```python
from build123d import *

# Parameters (mm, degrees)
F0_W     = 138.9888
F0_H     = 419.989
F1_DEPTH = 6.35
F3_D     = 7.874


with BuildPart() as f1:
    # F0 (on Top) → F1 (new body)
    with BuildSketch(Plane.XY):
        with Locations((69.4944, 309.9943)):
            Rectangle(F0_W, F0_H)
        Polygon((0, 619.9886), (0, 519.9888), (138.9888, 519.9888), (759.0028, 519.9888), (897.9916, 519.9888), (897.9916, 619.9886), align=None)
        with Locations((828.4972, 309.9943)):
            Rectangle(F0_W, F0_H)
        Polygon((0, 99.9998), (0, 0), (897.9916, 0), (897.9916, 99.9998), (759.0028, 99.9998), (138.9888, 99.9998), align=None)
    extrude(amount=F1_DEPTH)

    # F3 (through all)
    with Locations(Plane.XY.offset(6.35)):
        with Locations((108.9914, 539.9786), (124.0028, 554.99), (174.0154, 554.99), (124.0028, 579.9836), (224.028, 579.9836), (224.028, 554.99), (274.0406, 554.99), (324.0532, 579.9836), (324.0532, 554.99), (374.0658, 554.99), (424.0784, 579.9836), (424.0784, 554.99), (474.091, 579.9836), (474.091, 554.99), (524.1036, 554.99), (574.1162, 579.9836), (574.1162, 554.99), (624.1288, 554.99), (674.1414, 579.9836), (674.1414, 554.99), (789.0002, 539.9786), (774.1666, 579.9836), (774.1666, 554.99), (724.154, 554.99), (789.0002, 480.1108), (813.9938, 465.074), (789.0002, 130.0226), (813.9938, 145.034), (789.0002, 180.0352), (789.0002, 230.0478), (813.9938, 225.044), (789.0002, 280.0604), (813.9938, 305.054), (789.0002, 330.073), (789.0002, 380.0856), (813.9938, 385.064), (789.0002, 430.0982), (789.0002, 80.01), (774.1666, 64.9986), (774.1666, 40.005), (724.154, 64.9986), (674.1414, 64.9986), (674.1414, 40.005), (83.9978, 465.074), (108.9914, 480.1108), (108.9914, 430.0982), (83.9978, 385.064), (108.9914, 380.0856), (108.9914, 330.073), (83.9978, 305.054), (108.9914, 280.0604), (83.9978, 225.044), (108.9914, 230.0478), (108.9914, 180.0352), (83.9978, 145.034), (108.9914, 130.0226), (108.9914, 80.01), (124.0028, 64.9986), (124.0028, 40.005), (174.0154, 64.9986), (224.028, 40.005), (224.028, 64.9986), (274.0406, 64.9986), (324.0532, 40.005), (324.0532, 64.9986), (374.0658, 64.9986), (424.0784, 64.9986), (424.0784, 40.005), (474.091, 64.9986), (474.091, 40.005), (524.1036, 64.9986), (574.1162, 64.9986), (624.1288, 64.9986), (574.1162, 40.005)):
            Hole(F3_D / 2)


solid = f1.part
```
For this review, take the finished solid that the model builds, in its own axes (mm). Give positions to 0.01 mm unless a question says otherwise; leave off trailing zeros. Write each loop counter-clockwise with the first axis right and the second up, starting at its lowest first coordinate (ties: lowest second). Pieces come first, ordered by that corner, then holes.
Item 1: Insertion check: P1, Ø7, axis at x = 724.15, y = 65, coming from the -Z side. The pin has a flat end and moves straight along its axis. Give the tip position at first contact, or say it passes through.
Item 2: Wall thickness on probe 1 along X at (y, z) = (472.5, 3.5); probe 2 along Y at (x, z) = (201.5, 3); probe 3 along X at (y, z) = (542.5, 5.5): over which ranges is each line inside the solid? List them lowest first.
Item 3: Take a section at B-B (y = 110). Give the boundary of the cut face in (x, z).
Item 4: Take a section at C-C (z = 3). Give the number of separate pieces and of enclosed holes in the cut face, and give its area (3 significant figures).
Item 5: Take a section at A-A (x = 205). Give the boundary of the cut face in (y, z).
Established:
1. P1: passes through
2. probe 1: x = 0 to 138.99, 759 to 897.99
2. probe 2: y = 0 to 100, 519.99 to 619.99
2. probe 3: x = 0 to 105.97, 112.02 to 785.98, 792.02 to 897.99
3. outline: (0, 0) - (138.99, 0) - (138.99, 6.35) - (0, 6.35) - close; (759, 0) - (897.99, 0) - (897.99, 6.35) - (759, 6.35) - close
4. separate pieces: 1
4. enclosed holes: 75
4. area: 293,000 mm2
5. outline: (0, 0) - (100, 0) - (100, 6.35) - (0, 6.35) - close; (519.99, 0) - (619.99, 0) - (619.99, 6.35) - (519.99, 6.35) - close
